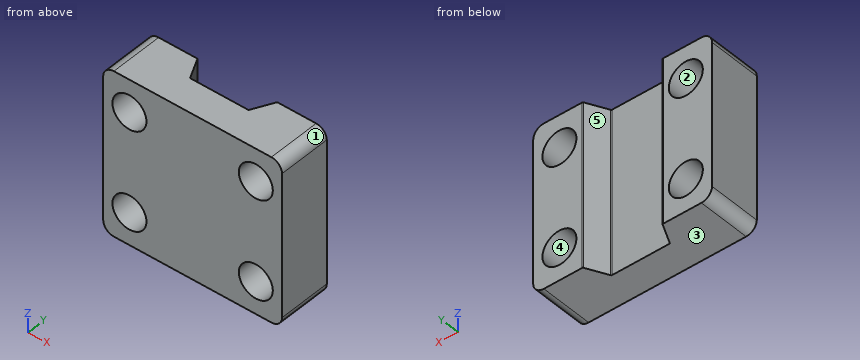
from build123d import *

# Parameters (mm, degrees)
SKETCH1_W               = 42.7228
SKETCH1_H               = 39.2176
SKETCH1_R               = 4.064
BOSS_EXTRUDE1_DEPTH     = 12.573
CUT_EXTRUDE1_DEPTH      = 1
CUT_EXTRUDE1_DEPTH_BACK = 40.2176
FILLET1_R               = 0.254
FILLET2_R               = 2.54


with BuildPart() as part:
    # Sketch1 → Boss-Extrude1 (new body)
    with BuildSketch(Plane(origin=(0, 0, 0), x_dir=(1, 0, 0), z_dir=(0, 1, 0))):
        Rectangle(SKETCH1_W, SKETCH1_H)
        with Locations((15.1003, -11.8745)):
            Circle(SKETCH1_R, mode=Mode.SUBTRACT)
        with Locations((-15.1003, 11.8745)):
            Circle(SKETCH1_R, mode=Mode.SUBTRACT)
        with Locations((15.1003, 11.8745)):
            Circle(SKETCH1_R, mode=Mode.SUBTRACT)
        with Locations((-15.1003, -11.8745)):
            Circle(SKETCH1_R, mode=Mode.SUBTRACT)
    extrude(amount=BOSS_EXTRUDE1_DEPTH)

    # Sketch2 → Cut-Extrude1 (cut, two sides)
    with BuildSketch(Plane.XY.offset(19.6088)) as cut_extrude1_sk:
        Polygon((-9.525, 12.573), (-6.985, 7.493), (6.985, 7.493), (9.525, 12.573), align=None)
    extrude(amount=CUT_EXTRUDE1_DEPTH, mode=Mode.SUBTRACT)
    extrude(cut_extrude1_sk.sketch, amount=-CUT_EXTRUDE1_DEPTH_BACK, mode=Mode.SUBTRACT)

    # Fillet1
    fillet1_edges = [part.edges().sort_by_distance(p)[0] for p in [
        (-9.525, 12.573, 0),
        (9.525, 12.573, 0),
        (6.985, 7.493, 0),
        (-6.985, 7.493, 0),
    ]]
    fillet(fillet1_edges, radius=FILLET1_R)

    # Fillet2
    fillet2_edges = [part.edges().sort_by_distance(p)[0] for p in [
        (21.3614, 6.2865, 19.6088),
        (-21.3614, 6.2865, 19.6088),
        (-21.3614, 6.2865, -19.6088),
        (21.3614, 6.2865, -19.6088),
    ]]
    fillet(fillet2_edges, radius=FILLET2_R)


solid = part.part
Could you check a few things on this model? Use its own coordinates, in mm. Face numbers are marked on the shaded views. A direction names the side the tool comes from. Give positions to 0.01 mm unless a question says otherwise; leave off trailing zeros. Order: outer loops, then holes, each group sorted by start corner. A loop starts at its lowest first (then second) coordinate and runs counter-clockwise, first axis right, second up. Notation, with made-up numbers: (49.5, 72.5) - (87.5, 72.5) arc R25 ccw to (87.5, 106.5) - close; hole circle Ø2 at (49, 46). An arc over 180 degrees is marked (long way). One line per item, written item: value. Start each with the question number.
1. Imagine slicing it at A-A on y = 9.75. List the corners of the cut face in (x, z) for me.
2. Thinking about a two-plate mould opening in Z: for the marked faces 1, 2 and 3, which applies, +Z half, -Z half, draft (parallel to the pull), parting line (faces both ways), or undercut?
3. For the marked faces 4 and 5, which set-ups out of +Z, -Z, +X, -X, +Y, -Y let a thin tool reach every point of the face, with its end or its side?
4. Imagine slicing it at B-B on z = 13. List the corners of the cut face in (x, y) for me, plus the area to 3 significant figures.
5. Imagine slicing it at C-C on x = -18. List the corners of the cut face in (y, z) for me, plus the area to 3 significant figures.
6. If I drill on probe 1 along X at (y, z) = (11.5, 12); probe 2 along Z at (x, y) = (14.5, 8.25); probe 3 along X at (y, z) = (9.75, -10), over which ranges is the centre line in solid material (lowest first)?
7. For P1, Ø12, axis at x = -5, z = 2, coming from the -Y side; P2, Ø4, axis at x = 3.5, z = 4, coming from the +Y side, each with a flat end and sliding along its axis, tell me the tip position at first contact or that it passes through.
8. Imagine slicing it at D-D on z = 4. List the corners of the cut face in (x, y) for me, plus the area to 3 significant figures.
Values:
1. outline: (-21.36, -17.07) arc R2.54 ccw to (-18.82, -19.61) - (-8.11, -19.61) - (-8.11, 19.61) - (-18.82, 19.61) arc R2.54 ccw to (-21.36, 17.07) - close; (8.11, -19.61) - (18.82, -19.61) arc R2.54 ccw to (21.36, -17.07) - (21.36, 17.07) arc R2.54 ccw to (18.82, 19.61) - (8.11, 19.61) - close; hole circle Ø8.13 at (-15.1, -11.87); hole circle Ø8.13 at (-15.1, 11.87); hole circle Ø8.13 at (15.1, -11.87); hole circle Ø8.13 at (15.1, 11.87)
2. face 1: +Z half
2. face 2: undercut
2. face 3: -Z half
3. face 4: +Y, -Y
3. face 5: +Z, -Z, +Y
4. outline: (-21.36, 0) - (-19.01, 0) - (-19.01, 12.57) - (-21.36, 12.57) - close; (-11.2, 0) - (11.2, 0) - (11.2, 12.57) - (9.68, 12.57) arc R0.25 ccw to (9.45, 12.43) - (7.06, 7.63) arc R0.25 cw to (6.83, 7.49) - (-6.83, 7.49) arc R0.25 cw to (-7.06, 7.63) - (-9.45, 12.43) arc R0.25 ccw to (-9.68, 12.57) - (-11.2, 12.57) - close; (19.01, 0) - (21.36, 0) - (21.36, 12.57) - (19.01, 12.57) - close
4. area: 257 mm²
5. outline: (0, -19.61) - (12.57, -19.61) - (12.57, -14.72) - (0, -14.72) - close; (0, -9.03) - (12.57, -9.03) - (12.57, 9.03) - (0, 9.03) - close; (0, 14.72) - (12.57, 14.72) - (12.57, 19.61) - (0, 19.61) - close
5. area: 350 mm²
6. probe 1: -21.36 to -19.16, -11.04 to -8.99, 8.99 to 11.04, 19.16 to 21.36
6. probe 2: -19.61 to -15.89, -7.86 to 7.86, 15.89 to 19.61
6. probe 3: -21.36 to -18.71, -11.49 to -8.11, 8.11 to 11.49, 18.71 to 21.36
7. P1: y = 0
7. P2: y = 7.49
8. outline: (-21.36, 0) - (21.36, 0) - (21.36, 12.57) - (9.68, 12.57) arc R0.25 ccw to (9.45, 12.43) - (7.06, 7.63) arc R0.25 cw to (6.83, 7.49) - (-6.83, 7.49) arc R0.25 cw to (-7.06, 7.63) - (-9.45, 12.43) arc R0.25 ccw to (-9.68, 12.57) - (-21.36, 12.57) - close
8. area: 453 mm²
